Here's how the part is built. I have some questions about the finished solid (model axes, mm). Face numbers are marked on the shaded views. A direction names the side the tool comes from. Round coordinates to 2 decimals unless told otherwise and drop trailing zeros. Loops run counter-clockwise (first coordinate to the right, second up) from the corner with the lowest first, then second, coordinate; pieces in that order, holes last. Notation, with made-up numbers: (-15.5, -13.75) - (31.5, -13.75) arc R34 cw to (31.5, 24.25) - close; hole circle Ø1 at (65.25, 36.25). An arc over 180 degrees is marked (long way). Answer as a JSON object with one key per item and string values. Group by question number.
1) Which directions (+Z, -Z, +X, -X, +Y, -Y) give clear straight access to the entire face, cutting with the end or side of a thin tool? Please do the marked faces 1, 2 and 3.
2) If we mould it in two halves opening along Y, with no side actions, what happens to the marked faces 4, 5, 6 and 7? For each: pulls with the +Y half, pulls with the -Y half, needs draft (parallel to the pull), parting line crosses it, or undercut.
3) I want a section at B-B, the plane y = 106.5. Please give me the cut outline in (x, z).
4) Will these pins go through, and if not, where does the flat tip stop? P1, Ø14, axis at x = 13.5, y = 104.5, coming from the -Z side; P2, Ø11, axis at x = 8, y = 39, coming from the -Z side; P3, Ø11, axis at x = 20, y = 28.5, coming from the -Z side; P4, Ø8, axis at x = 30.5, z = 9.5, coming from the -Y side.
5) I want a section at C-C, the plane y = 152. Please give me the cut outline in (x, z), then the cut area to 3 significant figures.
6) If I drill on line 1 along X through (y, z) = (44, 23.75); line 2 along Z through (x, y) = (23.5, 44.5); line 3 along X through (y, z) = (96.5, 5), over which ranges is the centre line in solid material (lowest first)? Write a range as [from, to].
7) I want a section at A-A, the plane z = 12. Give the number of separate pieces and of enclosed holes in the cut face, then the cut area to 3 significant figures.
8) I want a section at D-D, the plane y = 31.5. Please give me the cut outline in (x, z).
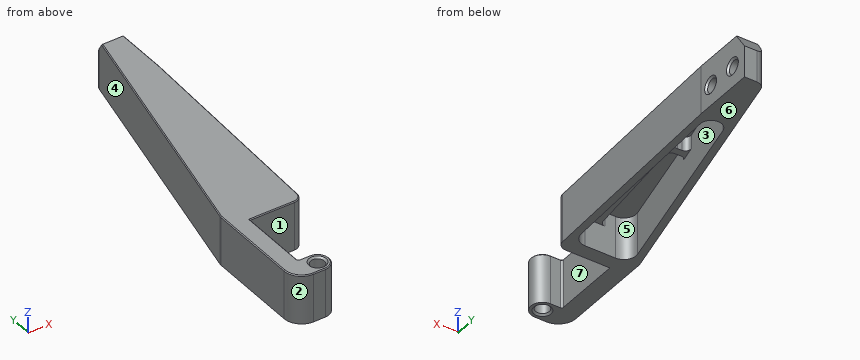
from build123d import *

# Parameters (mm, degrees)
SKETCH1_R           = 3.9
BOSS_EXTRUDE1_DEPTH = 28
SKETCH4_R           = 3.9
CUT_EXTRUDE2_DEPTH  = 10
CUT_EXTRUDE3_DEPTH  = 24
CHAMFER1_SIZE       = 1
CUT_EXTRUDE4_DEPTH  = 46
BOSS_EXTRUDE2_DEPTH = 8
FILLET1_R           = 3
CHAMFER2_SIZE       = 0.5


with BuildPart() as part:
    # Sketch1 → Boss-Extrude1 (new body)
    with BuildSketch(Plane.XY):
        with BuildLine():
            Line((6.7, -39.5), (1, -39.5))
            ThreePointArc((1, -39.5), (0.292893219, -39.207106781), (0, -38.5))
            Line((0, -38.5), (0, 0))
            Line((0, 0), (25.194477487, 0))
            ThreePointArc((25.194477487, 0), (28.659208118, 1.395053169), (30.190545371, 4.801743338))
            Line((30.190545371, 4.801743338), (35, 126))
            Line((35, 126), (35, 162))
            Line((35, 162), (28.005138809, 162))
            ThreePointArc((28.005138809, 162), (24.87921862, 160.902386831), (23.125718898, 158.091449191))
            Line((23.125718898, 158.091449191), (-9.879419911, 10.539063929))
            ThreePointArc((-9.879419911, 10.539063929), (-9.969763553, 9.996659567), (-10, 9.447614738))
            Line((-10, 9.447614738), (-10, -42.5))
            ThreePointArc((-10, -42.5), (-7.071067812, -49.571067812), (0, -52.5))
            Line((0, -52.5), (6.7, -52.5))
            ThreePointArc((6.7, -52.5), (13.2, -46), (6.7, -39.5))
        make_face()
        with Locations((6.7, -46)):
            Circle(SKETCH1_R, mode=Mode.SUBTRACT)
    extrude(amount=BOSS_EXTRUDE1_DEPTH)

    # Sketch4 → Cut-Extrude2 (cut)
    with BuildSketch(Plane(origin=(35, 0, 0), x_dir=(0, 0, -1), z_dir=(1, 0, 0))):
        with Locations((-12, 152)):
            Circle(SKETCH4_R)
        with Locations((-12, 134)):
            Circle(SKETCH4_R)
    extrude(amount=-CUT_EXTRUDE2_DEPTH, mode=Mode.SUBTRACT)

    # Sketch5 → Cut-Extrude3 (cut)
    with BuildSketch(Plane.XY):
        with BuildLine():
            Line((-4.440935128, 16.528028867), (18.877520205, 120.775240942))
            ThreePointArc((18.877520205, 120.775240942), (25.509806245, 125.414980777), (30.728105558, 119.227593919))
            Line((30.728105558, 119.227593919), (26.581075667, 14.722440673))
            ThreePointArc((26.581075667, 14.722440673), (24.437203514, 9.953074436), (19.58658063, 8))
            Line((19.58658063, 8), (2.390252747, 8))
            ThreePointArc((2.390252747, 8), (-3.073088816, 10.623711736), (-4.440935128, 16.528028867))
        make_face()
    extrude(amount=CUT_EXTRUDE3_DEPTH, mode=Mode.SUBTRACT)

    # Chamfer1
    chamfer1_edges = [part.edges().sort_by_distance(p)[0] for p in [
        (2.8, -46, 0),
        (2.8, -46, 28),
        (35, 152, 15.9),
        (35, 134, 15.9),
    ]]
    chamfer(chamfer1_edges, length=CHAMFER1_SIZE)

    # Sketch6 → Cut-Extrude4 (cut, through all)
    with BuildSketch(Plane(origin=(35, 0, 0), x_dir=(0, 0, -1), z_dir=(1, 0, 0))):
        Polygon((-18, 162), (-28, 154.997924618), (-28, 162), align=None)
    extrude(amount=-CUT_EXTRUDE4_DEPTH, mode=Mode.SUBTRACT)

    # Sketch7 → Boss-Extrude2 (add)
    with BuildSketch(Plane(origin=(0, 0, 24), x_dir=(-1, 0, 0), z_dir=(0, 0, -1))):
        with BuildLine():
            Line((-26.7218562, 119.256333807), (-22.401525887, 78.173226899))
            Line((-22.401525887, 78.173226899), (-29.088434109, 77.907873398))
            Line((-29.088434109, 77.907873398), (-28.929828779, 73.911019091))
            Line((-28.929828779, 73.911019091), (-21.982301269, 74.186714627))
            Line((-21.982301269, 74.186714627), (-15.022056754, 8))
            Line((-15.022056754, 8), (-11, 8))
            Line((-11, 8), (-17.976958991, 74.345656781))
            Line((-17.976958991, 74.345656781), (-8.575406865, 74.718734246))
            Line((-8.575406865, 74.718734246), (-9.462969579, 78.686661673))
            Line((-9.462969579, 78.686661673), (-18.396183609, 78.332169052))
            Line((-18.396183609, 78.332169052), (-22.743791996, 119.67467002))
            ThreePointArc((-22.743791996, 119.67467002), (-20.963928, 121.872870229), (-18.765727791, 120.093006233))
            ThreePointArc((-18.765727791, 120.093006233), (-25.360328417, 125.43259822), (-30.699920404, 118.837997594))
            ThreePointArc((-30.699920404, 118.837997594), (-28.920056409, 121.036197803), (-26.7218562, 119.256333807))
        make_face()
    extrude(amount=BOSS_EXTRUDE2_DEPTH)

    # Fillet1
    fillet1_edges = [part.edges().sort_by_distance(p)[0] for p in [
        (21.982301269, 74.186714627, 20),
        (15.022056754, 8, 20),
        (11, 8, 20),
        (17.976958991, 74.345656781, 20),
        (8.575406865, 74.718734246, 20),
        (9.462969579, 78.686661673, 20),
        (18.396183609, 78.332169052, 20),
        (22.401525887, 78.173226899, 20),
        (29.088434109, 77.907873398, 20),
        (28.929828779, 73.911019091, 20),
    ]]
    fillet(fillet1_edges, radius=FILLET1_R)

    # Chamfer2
    chamfer2_edges = [part.edges().sort_by_distance(p)[0] for p in [
        (32.595272685, 65.400871669, 28),
        (35, 140.498962309, 28),
        (-9.969763553, 9.996659567, 28),
        (-10, -16.526192631, 28),
        (-7.071067812, -49.571067812, 28),
        (3.35, -52.5, 28),
        (13.2, -46, 28),
        (12.597238744, 0, 28),
        (3.85, -39.5, 28),
        (0.292893219, -39.207106781, 28),
        (0, -19.25, 28),
        (28.659208118, 1.395053169, 28),
        (6.277163193, 82.768494273, 28),
    ]]
    chamfer(chamfer2_edges, length=CHAMFER2_SIZE)


solid = part.part
Outcome:
{
 "1": {"face 1": "+Z, -Z, +X", "face 2": "+Z, -Z, -X, -Y", "face 3": "-Z"},
 "2": {"face 4": "pulls with the +Y half", "face 5": "undercut", "face 6": "needs draft", "face 7": "undercut"},
 "3": {"outline": "(11.59, 0) - (15.68, 0) - (15.68, 24) - (21.36, 24) - (21.36, 16) - (25.38, 16) - (25.38, 24) - (30.22, 24) - (30.22, 0) - (34.23, 0) - (34.23, 27.5) - (33.73, 28) - (12.1, 28) - (11.59, 27.5) - close"},
 "4": {"P1": "z = 0", "P2": "z = 24", "P3": "z = 16", "P4": "y = 0.17"},
 "5": {"outline": "(21.76, 0) - (35, 0) - (35, 7.1) - (34, 8.1) - (25, 8.1) - (25, 15.9) - (34, 15.9) - (35, 16.9) - (35, 27.5) - (34.5, 28) - (22.28, 28) - (21.76, 27.5) - close", "area": "291 mm^2"},
 "6": {"line 1": "[-2.39, 1.7], [14.79, 18.81], [27.74, 31.75]", "line 2": "[24, 28]", "line 3": "[9.35, 13.45], [29.83, 33.83]"},
 "7": {"separate pieces": "1", "enclosed holes": "2", "area": "2,310 mm^2"},
 "8": {"outline": "(-5.19, 0) - (-1.09, 0) - (-1.09, 24) - (13.47, 24) - (13.47, 16) - (17.49, 16) - (17.49, 24) - (27.25, 24) - (27.25, 0) - (31.25, 0) - (31.25, 27.5) - (30.75, 28) - (-4.68, 28) - (-5.19, 27.5) - close"}
}
